The listing builds one solid part. Answer for the finished solid, in the listing's coordinates (mm). A direction names the side the tool comes from. Coordinates: 2 decimals unless noted, no trailing zeros. Write each loop counter-clockwise with the first axis right and the second up, starting at its lowest first coordinate (ties: lowest second). Pieces come first, ordered by that corner, then holes.
```python
from build123d import *

# Parameters (mm, degrees)
BOSS_EXTRUDE1_DEPTH = 1.524


with BuildPart() as part:
    # Sketch1 → Boss-Extrude1 (new body)
    with BuildSketch(Plane.XY):
        with BuildLine():
            Line((0, -11.304143944), (1.524, -11.304143944))
            Line((1.524, -11.304143944), (1.524, -8.333085901))
            ThreePointArc((1.524, -8.333085901), (3.945438138, -10.501523778), (4.87145261, -13.617287357))
            ThreePointArc((4.87145261, -13.617287357), (3.813444714, -17.660873454), (1.524, -21.157788112))
            ThreePointArc((1.524, -21.157788112), (-0.138732581, -21.765001835), (-1.77540365, -22.4393133))
            ThreePointArc((-1.77540365, -22.4393133), (-2.836636029, -23.830223279), (-2.99560227, -25.572513285))
            ThreePointArc((-2.99560227, -25.572513285), (-4.014612166, -24.876344883), (-4.669334398, -23.830223279))
            ThreePointArc((-4.669334398, -23.830223279), (-7.100142825, -25.212490369), (-9.437186958, -26.747976168))
            ThreePointArc((-9.437186958, -26.747976168), (-9.966611367, -27.75761792), (-10.13579223, -28.885024017))
            ThreePointArc((-10.13579223, -28.885024017), (-11.420458761, -28.850541305), (-12.64562455, -29.238518038))
            ThreePointArc((-12.64562455, -29.238518038), (-15.129726879, -31.532392213), (-17.428294378, -34.012152396))
            ThreePointArc((-17.428294378, -34.012152396), (-17.440615342, -34.566818357), (-16.992461897, -34.893872824))
            ThreePointArc((-16.992461897, -34.893872824), (-18.592932451, -36.063409356), (-20.055394787, -37.401514587))
            ThreePointArc((-20.055394787, -37.401514587), (-21.23200408, -39.175477677), (-22.32048354, -41.004840118))
            ThreePointArc((-22.32048354, -41.004840118), (-25.256637968, -43.106248561), (-28.366018586, -41.270854206))
            ThreePointArc((-28.366018586, -41.270854206), (-28.356027092, -41.137819843), (-28.345332967, -41.004840118))
            Line((-28.345332967, -41.004840118), (-25.899875794, -41.004840118))
            Line((-25.899875794, -41.004840118), (-25.899875794, -39.480840118))
            Line((-25.899875794, -39.480840118), (-28.171982443, -39.480840118))
            ThreePointArc((-28.171982443, -39.480840118), (-27.155881735, -35.169299836), (-25.402070376, -31.10162409))
            ThreePointArc((-25.402070376, -31.10162409), (-24.736304523, -28.780464694), (-24.763169881, -26.365862581))
            ThreePointArc((-24.763169881, -26.365862581), (-24.241136691, -27.302583764), (-23.389289994, -27.953984126))
            ThreePointArc((-23.389289994, -27.953984126), (-19.127839076, -23.515816288), (-13.919621322, -20.239878938))
            ThreePointArc((-13.919621322, -20.239878938), (-12.092421111, -18.838162319), (-10.781391169, -16.944839687))
            ThreePointArc((-10.781391169, -16.944839687), (-10.265088251, -18.039159093), (-9.174768374, -18.563855417))
            ThreePointArc((-9.174768374, -18.563855417), (-5.629295434, -17.960763676), (-2.03410657, -17.86740925))
            ThreePointArc((-2.03410657, -17.86740925), (-1.944710685, -14.656928393), (-2.99560227, -11.621997448))
            ThreePointArc((-2.99560227, -11.621997448), (-2.03410657, -9.489064634), (0, -8.333085901))
            Line((0, -8.333085901), (0, -11.304143944))
        make_face()
    extrude(amount=BOSS_EXTRUDE1_DEPTH)


solid = part.part
```
(1) Which of the six approach directions +Z, -Z, +X, -X, +Y, -Y give full straight-line access (tool end or side, diameter ignored) to faces 1 (the cylindrical face through (-7.067, -25.192, 0.751)), 2 (the cylindrical face through (-2.056, -9.514, 0.751)), 3 (the flat face through (-27, -39.481, 1)), 4 (the cylindrical face through (-24.25, -27.29, 0.75))?
(2) Find the intervals of material crossed by probe 1 along Y at (x, z) = (-2.5, 0.95); probe 2 along Y at (x, z) = (-24.5, 1.35); probe 3 along Y at (x, z) = (-11, 0.3), in increasing order.
(3) Section C-C, the plane x = -13.5 is taken. Write down the section's boundary in (y, z).
(4) For a pull along Y with two mould halves and no side action, classify faces 5 (the flat face through (-27, -41.005, 1)), 6 (the cylindrical face through (-12.115, -18.862, 0.751)), 7 (the flat face through (-13, -24, 1.524)) as pulls with the +Y half, pulls with the -Y half, needs draft (parallel to the pull), parting line crosses it, or undercut.
(5) Section B-B, the plane y = -30 is taken. Write down the section's boundary in (x, z), plus the area to 3 significant figures.
(6) Each of these flat-tipped pins is pushed along its axis until it touches: pin 1 (0.5 mm diameter, centred on x = 0.5, z = 0.5, fed in from +Y); pin 2 (0.8 mm diameter, centred on x = -27, z = 0.5, fed in from -Y); pin 3 (1 mm diameter, centred on x = -13, y = -30, fed in from -Z). Where does it stop, or does it pass through?
Solution:
1. face 1: +Z, -Z, -Y
1. face 2: +Z, -Z, -X, +Y
1. face 3: +Z, -Z, -X
1. face 4: +Z, -Z, +Y
2. probe 1: y = -23.19 to -17.85, -12.65 to -10.12
2. probe 2: y = -42.98 to -26.95
2. probe 3: y = -28.81 to -17.36
3. outline: (-29.99, 0) - (-19.99, 0) - (-19.99, 1.52) - (-29.99, 1.52) - close
4. face 5: undercut
4. face 6: pulls with the +Y half
4. face 7: needs draft
5. outline: (-24.99, 0) - (-13.51, 0) - (-13.51, 1.52) - (-24.99, 1.52) - close
5. area: 17.5 mm2
6. pin 1: stops at y = -11.3
6. pin 2: stops at y = -42.88
6. pin 3: stops at z = 0
